Read the model definition and answer for the solid it produces. Units are mm, in the model's axes. Face numbers are marked on the shaded views. A direction names the side the tool comes from. Round coordinates to 2 decimals unless told otherwise and drop trailing zeros. Order: outer loops, then holes, each group sorted by start corner. A loop starts at its lowest first (then second) coordinate and runs counter-clockwise, first axis right, second up. Notation, with made-up numbers: (56, 47.25) -> (91, 47.25) arc R37 cw to (91, 83.25) -> close; hole circle Ø4 at (9.5, 82). An arc over 180 degrees is marked (long way). Answer as a JSON object with one key per item and string values. Group by question number.
Item 1: Section A-A, the plane y = 101 is taken. Write down the section's boundary in (x, z).
Item 2: For the marked faces 1, 2 and 3, determine the directions among +Z, -Z, +X, -X, +Y, -Y from which every point of the face is accessible in a straight line to the end or side of a thin tool.
Item 3: Given P1, Ø4, axis at y = 34.5, z = -40, coming from the -X side; P2, Ø11.5, axis at x = 100.5, z = -38, coming from the +Y side; P3, Ø4, axis at x = 74, y = 17, coming from the -Z side, each flat-ended and moving along its own axis, determine where each tip first touches the part or whether it passes through.
Item 4: Section C-C, the plane z = -24 is taken. Write down the section's boundary in (x, y), plus the area to 4 significant figures.
Item 5: Section D-D, the plane x = -31 is taken. Write down the section's boundary in (y, z).
Item 6: Section B-B, the plane x = 126 is taken. Write down the section's boundary in (y, z), plus the area to 3 significant figures.
Item 7: Consider probe 1 along Y at (x, z) = (126, -6); probe 2 along Z at (x, y) = (110, 31); probe 3 along Y at (x, z) = (-62, -14). Determine where each line is inside the solid, lowest interval first. Write a range as from..to.
from build123d import *

# Parameters (mm, degrees)
BOSS_EXTRUDE2_DEPTH = 0.15
BOSS_EXTRUDE3_DEPTH = 0.00625
CUT_EXTRUDE2_REACH  = 2.202
SKETCH7_R           = 0.012
SCALE1_SCALE        = 1000


with BuildPart() as part:
    # Sketch4 → Boss-Extrude2 (new, symmetric)
    with BuildSketch(Plane(origin=(0, 0, 0), x_dir=(0, 0, -1), z_dir=(1, 0, 0))):
        Polygon((0, 0), (0, 0.125), (0.0125, 0.125), (0.0125, 0.0125), (0.05, 0.0125), (0.05, 0), align=None)
    extrude(amount=BOSS_EXTRUDE2_DEPTH, both=True)

    # Sketch6 → Boss-Extrude3 (add, symmetric)
    with BuildSketch(Plane(origin=(0, 0, 0), x_dir=(0, 0, -1), z_dir=(1, 0, 0))):
        Polygon((0.0125, 0.0125), (0.0125, 0.125), (0.05, 0.0125), align=None)
    extrude(amount=BOSS_EXTRUDE3_DEPTH, both=True)

    # Sketch7 → Cut-Extrude2 (cut, up to next)
    with BuildSketch(Plane.XY, mode=Mode.PRIVATE) as cut_extrude2_sk1:
        with Locations((-0.126, 0.101)):
            Circle(SKETCH7_R)
    cut_extrude2_tool1 = extrude(cut_extrude2_sk1.sketch, amount=-CUT_EXTRUDE2_REACH, mode=Mode.PRIVATE) & part.part
    cut_extrude2 = cut_extrude2_tool1.solids().sort_by_distance((-0.126, 0.101, 0))[0]
    add(cut_extrude2, mode=Mode.SUBTRACT)

    # Mirror1: Cut-Extrude2 across plane
    add(cut_extrude2.mirror(Plane(origin=(0, 0, 0), x_dir=(0, 0, 1), z_dir=(1, 0, 0))), mode=Mode.SUBTRACT)


with BuildPart() as part_1:
    # Scale1: scaled about (0, 0, 0)
    add(part.part.scale(SCALE1_SCALE))


solid = part_1.part
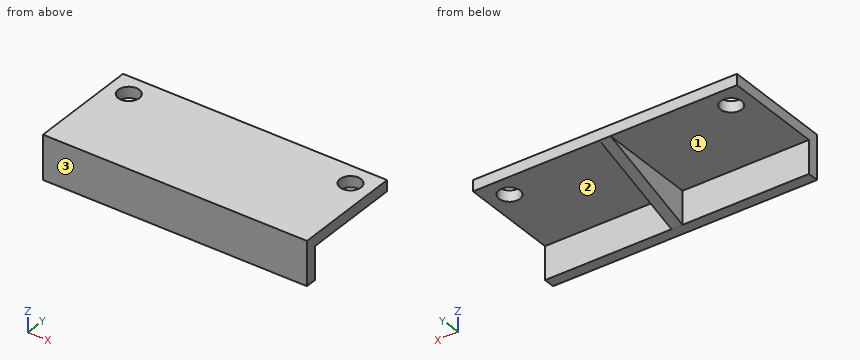
Values found:
{
 "1": {"outline": "(-150, -12.5) -> (-138, -12.5) -> (-138, 0) -> (-150, 0) -> close; (-114, -12.5) -> (-6.25, -12.5) -> (-6.25, -20.5) -> (6.25, -20.5) -> (6.25, -12.5) -> (114, -12.5) -> (114, 0) -> (-114, 0) -> close; (138, -12.5) -> (150, -12.5) -> (150, 0) -> (138, 0) -> close"},
 "2": {"face 1": "-Z, -X, +Y", "face 2": "-Z, +X, +Y", "face 3": "+Z, -Z, +X, -X, -Y"},
 "3": {"P1": "x = -6.25", "P2": "y = 12.5", "P3": "z = -12.5"},
 "4": {"outline": "(-150, 0) -> (150, 0) -> (150, 12.5) -> (6.25, 12.5) -> (6.25, 90.5) -> (-6.25, 90.5) -> (-6.25, 12.5) -> (-150, 12.5) -> close", "area": "4,725 mm2"},
 "5": {"outline": "(0, -50) -> (12.5, -50) -> (12.5, -12.5) -> (125, -12.5) -> (125, 0) -> (0, 0) -> close"},
 "6": {"outline": "(0, -50) -> (12.5, -50) -> (12.5, -12.5) -> (89, -12.5) -> (89, 0) -> (0, 0) -> close; (113, -12.5) -> (125, -12.5) -> (125, 0) -> (113, 0) -> close", "area": "1,730 mm2"},
 "7": {"probe 1": "0..89, 113..125", "probe 2": "-12.5..0", "probe 3": "0..12.5"}
}
